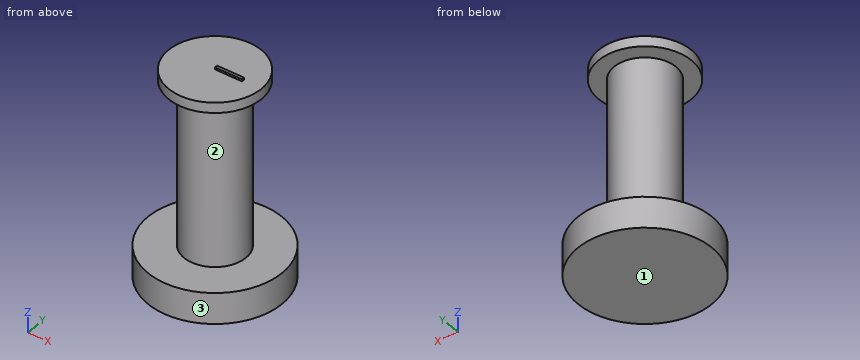
```python
from build123d import *

# Parameters (mm, degrees)
SKETCH_1_R          = 80
EXTRUDE_1_DEPTH     = 30
SKETCH_2_R          = 30
EXTRUDE_2_DEPTH     = 160
SKETCH_3_R          = 45
EXTRUDE_3_DEPTH     = 10
SKETCH_5_W          = 26.757416482
SKETCH_5_H          = 2.773634635
EXTRUDE_6_DEPTH     = 2
SKETCH_6_R          = 97.779490514
SKETCH_6_R_2        = 65
CUT_EXTRUDE_1_DEPTH = 42
SCALE_2_SCALE       = 0.345


with BuildPart() as part:
    # 草图1 → 凸台-拉伸1 (new body)
    with BuildSketch(Plane.XY):
        Circle(SKETCH_1_R)
    extrude(amount=EXTRUDE_1_DEPTH)

    # 草图2 → 凸台-拉伸2 (add)
    with BuildSketch(Plane.XY.offset(30)):
        Circle(SKETCH_2_R)
    extrude(amount=EXTRUDE_2_DEPTH)

    # 草图3 → 凸台-拉伸3 (add)
    with BuildSketch(Plane.XY.offset(190)):
        Circle(SKETCH_3_R)
    extrude(amount=EXTRUDE_3_DEPTH)

    # 草图5 → 凸台-拉伸6 (add)
    with BuildSketch(Plane.XY.offset(200)):
        with Locations((13.378708241, 1.386817318)):
            Rectangle(SKETCH_5_W, SKETCH_5_H)
    extrude(amount=EXTRUDE_6_DEPTH)

    # 草图6 → 切除-拉伸1 (cut)
    with BuildSketch(Plane(origin=(0, 0, 0), x_dir=(-1, 0, 0), z_dir=(0, 0, -1))):
        Circle(SKETCH_6_R)
        Circle(SKETCH_6_R_2, mode=Mode.SUBTRACT)
    extrude(amount=-CUT_EXTRUDE_1_DEPTH, mode=Mode.SUBTRACT)


with BuildPart() as part_1:
    # 缩放比例2: scaled about (0, 0, 0)
    add(part.part.scale(SCALE_2_SCALE))


solid = part_1.part
```
Work out the finished part from the listing and answer in its coordinate system (mm). Face numbers are marked on the shaded views. Coordinates: 2 decimals unless noted, no trailing zeros. Loops run counter-clockwise (first coordinate to the right, second up) from the corner with the lowest first, then second, coordinate; pieces in that order, holes last.
1) Section A-A (y = -12.5) is taken. Give the vertices of the cut face in (x, z), plus the area to 3 significant figures.
Results:
outline: (-18.62, 0) - (18.62, 0) - (18.62, 10.35) - (-18.62, 10.35) - close; (-9.21, 65.55) - (9.21, 65.55) - (9.21, 69) - (-9.21, 69) - close
area: 449 mm2
2) Flat-ended cylindrical pins translate along their axes: pin 1 (10 mm diameter, centred on x = -1.5, z = 24.5, fed in from -Y); pin 2 (2 mm diameter, centred on y = -10.5, z = 60.5, fed in from +X); pin 3 (5 mm diameter, centred on y = -1.5, z = 15.5, fed in from -X); pin 4 (6 mm diameter, centred on y = 15, z = 34.5, fed in from +X). Find the tip coordinate at first contact, or state that the pin passes through.
Results:
pin 1: stops at y = -10.35
pin 2: stops at x = 4.11
pin 3: stops at x = -10.35
pin 4: passes through
3) Section D-D (z = 33) is taken. Give the vertices of the cut face in (x, y).
Results:
outline: circle Ø20.7 at (0, 0)
4) Section B-B (x = 13) is taken. Give the vertices of the cut face in (y, z).
Results:
outline: (-18.27, 0) - (18.27, 0) - (18.27, 10.35) - (-18.27, 10.35) - close; (-8.49, 65.55) - (8.49, 65.55) - (8.49, 69) - (-8.49, 69) - close
5) Section C-C (x = -2) is taken. Give the vertices of the cut face in (y, z).
Results:
outline: (-22.34, 0) - (22.34, 0) - (22.34, 10.35) - (10.15, 10.35) - (10.15, 65.55) - (15.4, 65.55) - (15.4, 69) - (-15.4, 69) - (-15.4, 65.55) - (-10.15, 65.55) - (-10.15, 10.35) - (-22.34, 10.35) - close
6) Consider probe 1 along Z at (x, y) = (-12.5, 8.5); probe 2 along Y at (x, z) = (0, 31.5); probe 3 along Z at (x, y) = (-19, 9.5). Determine where each line is inside the solid, lowest interval first.
Results:
probe 1: z = 0 to 10.35, 65.55 to 69
probe 2: y = -10.35 to 10.35
probe 3: z = 0 to 10.35
7) For a pull along Z with two mould halves and no side action, classify the marked faces 1, 2 and 3 as +Z half, -Z half, draft (parallel to the pull), parting line (faces both ways), or undercut.
Results:
face 1: -Z half
face 2: undercut
face 3: draft
